Verification items for the finished model (mm, model axes). A direction names the side the tool comes from. Round coordinates to 2 decimals unless told otherwise and drop trailing zeros. Order: outer loops, then holes, each group sorted by start corner. A loop starts at its lowest first (then second) coordinate and runs counter-clockwise, first axis right, second up. Notation, with made-up numbers: M -24.5,4.5 L 24.5,4.5 A28 cw 24.5,33.5 Z; hole C 13,-6.5 d11. An arc over 180 degrees is marked long. Use one line per item in the form item = value. Start each with the question number.
Item 1: Thickness scan on probe 1 along X at (y, z) = (2, 65); probe 2 along Z at (x, y) = (86.5, 0.6); probe 3 along X at (y, z) = (-1, 42). Record the ranges inside material, lowest first. Write a range as [from, to].
Item 2: Cross-section at B-B on z = -16. Enter the section's corners in (x, y), then the cut area to 3 significant figures.
Item 3: Release check for a two-part mould opening along Y. For faces 4 (the flat face through (49, -3, -15)), 5 (the flat face through (31, -20, 0)), 6 (the flat face through (91.5, -2.8, -15.2)) record: +Y half, -Y half, draft (parallel to the pull), parting line (faces both ways), or undercut.
Item 4: Cross-section at D-D on x = 26.5. Enter the section's corners in (y, z), then the cut area to 3 significant figures.
Item 5: Go/stop test with flat-tipped pins: pin 1 Ø8 at (x, z) = (72.5, -48) entering from -Y; pin 2 Ø12 at (x, z) = (39.5, 17.5) entering from -Y; pin 3 Ø12 at (x, y) = (60.5, -11.5) entering from -Z. Record where each tip stops, or that it passes through.
Item 6: Cross-section at C-C on x = -29. Enter the section's corners in (y, z), then the cut area to 3 significant figures.
Item 7: Cross-section at A-A on z = -30. Enter the section's corners in (x, y).
Item 8: Tool access check on faces 1 (the flat face through (52, -17.15, 16)), 2 (the flat face through (51, 0, -46)), 3 (the flat face through (51, -3, 15)). Record the directions out of +Z, -Z, +X, -X, +Y, -Y that give a thin tool (end or side, any length) a straight path to the whole face; none if there is none.
from build123d import *

# Parameters (mm, degrees)
SKETCH1_W               = 183
SKETCH1_H               = 140
BOSS_EXTRUDE1_DEPTH     = 3
SKETCH2_W               = 78
SKETCH2_H               = 140
BOSS_EXTRUDE2_DEPTH     = 30
SKETCH3_W               = 72
SKETCH3_H               = 30
CUT_EXTRUDE1_DEPTH      = 140
SKETCH5_W               = 80
SKETCH5_H               = 70
BOSS_EXTRUDE3_DEPTH     = 25
CUT_EXTRUDE2_DEPTH      = 199.214530244
CUT_EXTRUDE2_DEPTH_BACK = 85
SKETCH7_W               = 20
SKETCH7_H               = 30
CUT_EXTRUDE3_DEPTH      = 85
SKETCH8_W               = 60
SKETCH8_H               = 20
CUT_EXTRUDE4_DEPTH      = 85
SKETCH9_W               = 50
SKETCH9_H               = 15
CUT_EXTRUDE5_DEPTH      = 10
SKETCH11_W              = 20
SKETCH11_H              = 20
CUT_EXTRUDE6_DEPTH      = 10
SKETCH12_W              = 20
SKETCH12_H              = 20
CUT_EXTRUDE7_DEPTH      = 10
SKETCH15_W              = 42
SKETCH15_H              = 100
CUT_EXTRUDE8_DEPTH      = 10
SKETCH16_W              = 13.088467217
SKETCH16_H              = 23
BOSS_EXTRUDE4_DEPTH     = 83
SKETCH17_W              = 13.301151585
SKETCH17_H              = 23.738473688
BOSS_EXTRUDE5_DEPTH     = 83
SKETCH18_W              = 83
SKETCH18_H              = 6
BOSS_EXTRUDE6_DEPTH     = 8
SKETCH19_W              = 83
SKETCH19_H              = 6
BOSS_EXTRUDE7_DEPTH     = 8
SKETCH20_W              = 14
SKETCH20_H              = 25
CUT_EXTRUDE9_DEPTH      = 80
SKETCH21_W              = 14
SKETCH21_H              = 25
CUT_EXTRUDE10_DEPTH     = 80
SKETCH22_W              = 42
SKETCH22_H              = 3
CUT_EXTRUDE11_DEPTH     = 80
SKETCH23_W              = 10
SKETCH23_H              = 100
CUT_EXTRUDE12_DEPTH     = 3
SKETCH24_W              = 80.000727439
SKETCH24_H              = 8
CUT_EXTRUDE13_DEPTH     = 3
SKETCH25_W              = 11
SKETCH25_H              = 4.85
BOSS_EXTRUDE9_DEPTH     = 83
SKETCH26_W              = 11
SKETCH26_H              = 4.85
BOSS_EXTRUDE10_DEPTH    = 83
SKETCH27_W              = 11
SKETCH27_H              = 4.85
CUT_EXTRUDE14_DEPTH     = 80
SKETCH28_W              = 11
SKETCH28_H              = 4.85
CUT_EXTRUDE15_DEPTH     = 80
SKETCH29_W              = 15
SKETCH29_H              = 27
CUT_EXTRUDE16_DEPTH     = 12
FILLET2_R               = 1
SKETCH30_R              = 1.5
CUT_EXTRUDE17_DEPTH     = 3
SKETCH31_R              = 1.5
CUT_EXTRUDE18_DEPTH     = 3
SKETCH32_R              = 1.5
CUT_EXTRUDE19_DEPTH     = 3
SKETCH33_R              = 1.5
CUT_EXTRUDE20_DEPTH     = 3


with BuildPart() as part:
    # Sketch1 → Boss-Extrude1 (new body)
    with BuildSketch(Plane(origin=(0, 0, 0), x_dir=(1, 0, 0), z_dir=(0, 1, 0))):
        Rectangle(SKETCH1_W, SKETCH1_H)
    extrude(amount=BOSS_EXTRUDE1_DEPTH)

    # Sketch2 → Boss-Extrude2 (add)
    with BuildSketch(Plane.XZ):
        with Locations((-27.5, 0)):
            Rectangle(SKETCH2_W, SKETCH2_H)
    extrude(amount=BOSS_EXTRUDE2_DEPTH)

    # Sketch3 → Cut-Extrude1 (cut)
    with BuildSketch(Plane.XY.offset(70)):
        with Locations((-27.5, -12)):
            Rectangle(SKETCH3_W, SKETCH3_H)
    extrude(amount=-CUT_EXTRUDE1_DEPTH, mode=Mode.SUBTRACT)

    # Sketch5 → Boss-Extrude3 (add)
    with BuildSketch(Plane.XZ):
        with Locations((51.5, 0)):
            Rectangle(SKETCH5_W, SKETCH5_H)
    extrude(amount=BOSS_EXTRUDE3_DEPTH)

    # Sketch6 → Cut-Extrude2 (cut, two sides: drawn at the far end of the back side and taken through both)
    with BuildSketch(Plane(origin=(91.5, 0, 0), x_dir=(0, 0, -1), z_dir=(1, 0, 0)).offset(-CUT_EXTRUDE2_DEPTH_BACK)):
        Polygon((-20, 204.718543704), (-20, 3), (-20, -4.67262363), (-30, -4.67262363), (-30, -20), (30, -20), (30, -4.67262363), (20, -4.67262363), (20, 3), (20, 204.718543704), (20, 608.155631112), (-20, 608.155631112), align=None)
    extrude(amount=CUT_EXTRUDE2_DEPTH + CUT_EXTRUDE2_DEPTH_BACK, mode=Mode.SUBTRACT)

    # Sketch7 → Cut-Extrude3 (cut)
    with BuildSketch(Plane(origin=(0, -27, 0), x_dir=(1, 0, 0), z_dir=(0, 1, 0))):
        with Locations((-18.5, 10)):
            Rectangle(SKETCH7_W, SKETCH7_H)
    extrude(amount=-CUT_EXTRUDE3_DEPTH, mode=Mode.SUBTRACT)

    # Sketch8 → Cut-Extrude4 (cut)
    with BuildSketch(Plane(origin=(-63.5, 0, 0), x_dir=(0, 0, -1), z_dir=(1, 0, 0))):
        with Locations((10, -12)):
            Rectangle(SKETCH8_W, SKETCH8_H)
    extrude(amount=-CUT_EXTRUDE4_DEPTH, mode=Mode.SUBTRACT)

    # Sketch9 → Cut-Extrude5 (cut)
    with BuildSketch(Plane.XZ.offset(25)):
        with Locations((56.5, 0)):
            Rectangle(SKETCH9_W, SKETCH9_H)
    extrude(amount=-CUT_EXTRUDE5_DEPTH, mode=Mode.SUBTRACT)

    # Sketch11 → Cut-Extrude6 (cut)
    with BuildSketch(Plane(origin=(-63.5, 0, 0), x_dir=(0, 0, -1), z_dir=(1, 0, 0))):
        with Locations((-30, -12)):
            Rectangle(SKETCH11_W, SKETCH11_H)
    extrude(amount=-CUT_EXTRUDE6_DEPTH, mode=Mode.SUBTRACT)

    # Sketch12 → Cut-Extrude7 (cut)
    with BuildSketch(Plane(origin=(0, -27, 0), x_dir=(1, 0, 0), z_dir=(0, 1, 0))):
        with Locations((-18.5, -15)):
            Rectangle(SKETCH12_W, SKETCH12_H)
    extrude(amount=-CUT_EXTRUDE7_DEPTH, mode=Mode.SUBTRACT)

    # Sketch15 → Cut-Extrude8 (cut)
    with BuildSketch(Plane(origin=(0, -27, 0), x_dir=(1, 0, 0), z_dir=(0, 1, 0))):
        with Locations((-32.5, 0)):
            Rectangle(SKETCH15_W, SKETCH15_H)
    extrude(amount=-CUT_EXTRUDE8_DEPTH, mode=Mode.SUBTRACT)

    # Sketch16 → Boss-Extrude4 (add)
    with BuildSketch(Plane(origin=(91.5, 0, 0), x_dir=(0, 0, -1), z_dir=(1, 0, 0))):
        with Locations((-25.544233609, -8.5)):
            Rectangle(SKETCH16_W, SKETCH16_H)
    extrude(amount=-BOSS_EXTRUDE4_DEPTH)

    # Sketch17 → Boss-Extrude5 (add)
    with BuildSketch(Plane(origin=(91.5, 0, 0), x_dir=(0, 0, -1), z_dir=(1, 0, 0))):
        with Locations((25.650575792, -8.869236844)):
            Rectangle(SKETCH17_W, SKETCH17_H)
    extrude(amount=-BOSS_EXTRUDE5_DEPTH)

    # Sketch18 → Boss-Extrude6 (add)
    with BuildSketch(Plane(origin=(0, 0, 19), x_dir=(-1, 0, 0), z_dir=(0, 0, -1))):
        with Locations((-50, 0)):
            Rectangle(SKETCH18_W, SKETCH18_H)
    extrude(amount=BOSS_EXTRUDE6_DEPTH)

    # Sketch19 → Boss-Extrude7 (add)
    with BuildSketch(Plane.XY.offset(-19)):
        with Locations((50, 0)):
            Rectangle(SKETCH19_W, SKETCH19_H)
    extrude(amount=BOSS_EXTRUDE7_DEPTH)

    # Sketch20 → Cut-Extrude9 (cut)
    with BuildSketch(Plane(origin=(91.5, 0, 0), x_dir=(0, 0, -1), z_dir=(1, 0, 0))):
        with Locations((-28, -12.5)):
            Rectangle(SKETCH20_W, SKETCH20_H)
    extrude(amount=-CUT_EXTRUDE9_DEPTH, mode=Mode.SUBTRACT)

    # Sketch21 → Cut-Extrude10 (cut)
    with BuildSketch(Plane(origin=(91.5, 0, 0), x_dir=(0, 0, -1), z_dir=(1, 0, 0))):
        with Locations((28, -12.5)):
            Rectangle(SKETCH21_W, SKETCH21_H)
    extrude(amount=-CUT_EXTRUDE10_DEPTH, mode=Mode.SUBTRACT)

    # Sketch22 → Cut-Extrude11 (cut)
    with BuildSketch(Plane(origin=(91.5, 0, 0), x_dir=(0, 0, -1), z_dir=(1, 0, 0))):
        with Locations((0, -23.5)):
            Rectangle(SKETCH22_W, SKETCH22_H)
    extrude(amount=-CUT_EXTRUDE11_DEPTH, mode=Mode.SUBTRACT)

    # Sketch23 → Cut-Extrude12 (cut)
    with BuildSketch(Plane(origin=(0, -27, 0), x_dir=(1, 0, 0), z_dir=(0, 1, 0))):
        with Locations((-58.5, 0)):
            Rectangle(SKETCH23_W, SKETCH23_H)
    extrude(amount=-CUT_EXTRUDE12_DEPTH, mode=Mode.SUBTRACT)

    # Sketch24 → Cut-Extrude13 (cut)
    with BuildSketch(Plane(origin=(-63.5, 0, 0), x_dir=(0, 0, -1), z_dir=(1, 0, 0))):
        with Locations((0.00036372, -26)):
            Rectangle(SKETCH24_W, SKETCH24_H)
    extrude(amount=-CUT_EXTRUDE13_DEPTH, mode=Mode.SUBTRACT)

    # Sketch25 → Boss-Extrude9 (add)
    with BuildSketch(Plane(origin=(91.5, 0, 0), x_dir=(0, 0, -1), z_dir=(1, 0, 0))):
        with Locations((-13.5, -17.575)):
            Rectangle(SKETCH25_W, SKETCH25_H)
    extrude(amount=-BOSS_EXTRUDE9_DEPTH)

    # Sketch26 → Boss-Extrude10 (add)
    with BuildSketch(Plane(origin=(91.5, 0, 0), x_dir=(0, 0, -1), z_dir=(1, 0, 0))):
        with Locations((13.5, -17.575)):
            Rectangle(SKETCH26_W, SKETCH26_H)
    extrude(amount=-BOSS_EXTRUDE10_DEPTH)

    # Sketch27 → Cut-Extrude14 (cut)
    with BuildSketch(Plane(origin=(91.5, 0, 0), x_dir=(0, 0, -1), z_dir=(1, 0, 0))):
        with Locations((-15.5, -19.575)):
            Rectangle(SKETCH27_W, SKETCH27_H)
    extrude(amount=-CUT_EXTRUDE14_DEPTH, mode=Mode.SUBTRACT)

    # Sketch28 → Cut-Extrude15 (cut)
    with BuildSketch(Plane(origin=(91.5, 0, 0), x_dir=(0, 0, -1), z_dir=(1, 0, 0))):
        with Locations((15.5, -19.575)):
            Rectangle(SKETCH28_W, SKETCH28_H)
    extrude(amount=-CUT_EXTRUDE15_DEPTH, mode=Mode.SUBTRACT)

    # Sketch29 → Cut-Extrude16 (cut)
    with BuildSketch(Plane(origin=(0, 3, 0), x_dir=(1, 0, 0), z_dir=(0, 1, 0))):
        with Locations((47.741795072, -46.5)):
            Rectangle(SKETCH29_W, SKETCH29_H)
    extrude(amount=-CUT_EXTRUDE16_DEPTH, mode=Mode.SUBTRACT)

    # Fillet2
    fillet2_edges = [part.edges().sort_by_distance(p)[0] for p in [
        (91.5, 3, 40.5),
        (50, 3, -70),
        (50, 3, 70),
        (-77.5, 3, -70),
        (-63.5, 3, 0),
        (8.5, 3, -40.5),
        (-91.5, 3, 0),
        (8.5, 3, 40.5),
        (91.5, 3, -40.5),
        (-77.5, 3, 70),
    ]]
    fillet(fillet2_edges, radius=FILLET2_R)

    # Sketch30 → Cut-Extrude17 (cut)
    with BuildSketch(Plane(origin=(0, 3, 0), x_dir=(1, 0, 0), z_dir=(0, 1, 0))):
        with Locations(Location((-86.5, -65, 0), (0, 0, 270))):
            Circle(SKETCH30_R)
    extrude(amount=-CUT_EXTRUDE17_DEPTH, mode=Mode.SUBTRACT)

    # Sketch31 → Cut-Extrude18 (cut)
    with BuildSketch(Plane(origin=(0, 3, 0), x_dir=(1, 0, 0), z_dir=(0, 1, 0))):
        with Locations(Location((-86.5, 65, 0), (0, 0, 270))):
            Circle(SKETCH31_R)
    extrude(amount=-CUT_EXTRUDE18_DEPTH, mode=Mode.SUBTRACT)

    # Sketch32 → Cut-Extrude19 (cut)
    with BuildSketch(Plane(origin=(0, 3, 0), x_dir=(1, 0, 0), z_dir=(0, 1, 0))):
        with Locations(Location((86.5, 65, 0), (0, 0, 270))):
            Circle(SKETCH32_R)
    extrude(amount=-CUT_EXTRUDE19_DEPTH, mode=Mode.SUBTRACT)

    # Sketch33 → Cut-Extrude20 (cut)
    with BuildSketch(Plane(origin=(0, 3, 0), x_dir=(1, 0, 0), z_dir=(0, 1, 0))):
        with Locations(Location((86.5, -65, 0), (0, 0, 270))):
            Circle(SKETCH33_R)
    extrude(amount=-CUT_EXTRUDE20_DEPTH, mode=Mode.SUBTRACT)


solid = part.part
Output values:
q1.probe_1 = [-91.5, -88], [-85, -63.5], [8.5, 85], [88, 91.5]
q1.probe_2 = [-70, -66.5], [-63.5, -11], [11, 63.5], [66.5, 70]
q1.probe_3 = [-66.5, -63.5], [8.5, 11.5]
q2.outline = M -91.5,0 L -66.5,0 L -66.5,-2 L -63.5,-2 L -63.5,2 A1 ccw -64.5,3 L -90.5,3 A1 ccw -91.5,2 Z; M -8.5,-30 L 11.5,-30 L 11.5,-17.15 L 91.5,-17.15 L 91.5,-15.15 L 8.5,-15.15 L 8.5,-27 L -8.5,-27 Z; M 8.5,-3 L 91.5,-3 L 91.5,2 A1 ccw 90.5,3 L 9.5,3 A1 ccw 8.5,2 Z
q2.area = 843 mm2
q3.face_4 = undercut
q3.face_5 = +Y half
q3.face_6 = draft
q4.outline = M -22,-10 L -17.15,-10 L -17.15,-21 L 0,-21 L 0,-70 L 2,-70 A1 ccw 3,-69 L 3,-11 L -3,-11 L -3,-19 L -15.15,-19 L -15.15,-8 L -20,-8 L -20,8 L -15.15,8 L -15.15,19 L -3,19 L -3,11 L 3,11 L 3,69 A1 ccw 2,70 L 0,70 L 0,21 L -17.15,21 L -17.15,10 L -22,10 Z
q4.area = 566 mm2
q5.pin_1 = 0
q5.pin_2 = -17.15
q5.pin_3 = -21
q6.outline = M -30,-70 L -27,-70 L -27,-50 L -30,-50 Z; M -30,50 L -27,50 L -27,70 L -30,70 Z
q6.area = 120 mm2
q7.outline = M -91.5,0 L -66.5,0 L -66.5,-2 L -63.5,-2 L -63.5,2 A1 ccw -64.5,3 L -90.5,3 A1 ccw -91.5,2 Z; M -11.5,-30 L 11.5,-30 L 11.5,0 L 91.5,0 L 91.5,2 A1 ccw 90.5,3 L 9.5,3 A1 ccw 8.5,2 L 8.5,-27 L -11.5,-27 Z
q8.face_1 = +Z, +X, -Y
q8.face_2 = -Z, +X, -Y
q8.face_3 = +X, -X
